Model file for the job. Use its own axes, mm. A direction names the side the tool comes from. Give positions to 0.01 mm unless a question says otherwise; leave off trailing zeros. Loops run counter-clockwise (first coordinate to the right, second up) from the corner with the lowest first, then second, coordinate; pieces in that order, holes last. Notation, with made-up numbers: M 81.25,45.5 L 134.25,45.5 A12 cw 134.25,66.5 Z; hole C 35.5,51.25 d8. An arc over 180 degrees is marked long. Answer in a Markdown table with one row per item.
```python
from build123d import *

# Parameters (mm, degrees)
SKETCH1_R           = 3.1
BOSS_EXTRUDE4_DEPTH = 13.7
SKETCH6_W           = 24.96
SKETCH6_H           = 31.16
CUT_EXTRUDE1_DEPTH  = 12.5
SKETCH7_W           = 19.96
SKETCH7_H           = 26.16
CUT_EXTRUDE2_DEPTH  = 12.5
SKETCH9_W           = 1.2
SKETCH9_H           = 12.5
CUT_EXTRUDE3_DEPTH  = 1.45
SKETCH10_W          = 1.2
SKETCH10_H          = 12.5
CUT_EXTRUDE4_DEPTH  = 1.45
CUT_EXTRUDE5_DEPTH  = 1.5
SKETCH12_W          = 7.5
SKETCH12_H          = 6
CUT_EXTRUDE6_DEPTH  = 20.892135624
BOSS_EXTRUDE5_DEPTH = 6
BOSS_EXTRUDE6_DEPTH = 7.7


with BuildPart() as part:
    # Sketch1 → Boss-Extrude4 (new body)
    with BuildSketch(Plane(origin=(0, 0, 0), x_dir=(1, 0, 0), z_dir=(0, 1, 0))):
        with BuildLine():
            Line((-1.559985024, 16.088570711), (-23.661955043, 33.271658997))
            ThreePointArc((-23.661955043, 33.271658997), (-29.74307331, 33.27087194), (-29.742286254, 27.189753673))
            Line((-29.742286254, 27.189753673), (-12.559985024, 5.088570711))
            Line((-12.559985024, 5.088570711), (-12.559985024, -6.971429289))
            Line((-12.559985024, -6.971429289), (-29.742286254, -29.072612251))
            ThreePointArc((-29.742286254, -29.072612251), (-29.74307331, -35.153730518), (-23.661955043, -35.154517574))
            Line((-23.661955043, -35.154517574), (-1.559985024, -17.971429289))
            Line((-1.559985024, -17.971429289), (4.300014976, -17.971429289))
            Line((4.300014976, -17.971429289), (26.401984994, -35.154517574))
            ThreePointArc((26.401984994, -35.154517574), (32.483103261, -35.153730518), (32.482316205, -29.072612251))
            Line((32.482316205, -29.072612251), (15.300014976, -6.971429289))
            Line((15.300014976, -6.971429289), (15.300014976, 5.088570711))
            Line((15.300014976, 5.088570711), (32.482316205, 27.189753673))
            ThreePointArc((32.482316205, 27.189753673), (32.483103261, 33.27087194), (26.401984994, 33.271658997))
            Line((26.401984994, 33.271658997), (4.300014976, 16.088570711))
            Line((4.300014976, 16.088570711), (-1.559985024, 16.088570711))
        make_face()
        with BuildLine():
            Line((15.300014976, -17.971429289), (15.300014976, -8.926547914))
            Line((15.300014976, -8.926547914), (30.013101167, -27.851638652))
            ThreePointArc((30.013101167, -27.851638652), (26.40152787, -29.073069325), (25.180248217, -32.684693693))
            Line((25.180248217, -32.684693693), (6.255121178, -17.971429289))
            Line((6.255121178, -17.971429289), (15.300014976, -17.971429289))
        make_face(mode=Mode.SUBTRACT)
        with Locations((-26.702120648, -32.113564912)):
            Circle(SKETCH1_R, mode=Mode.SUBTRACT)
        with BuildLine():
            Line((-12.559985024, -8.926547914), (-12.559985024, -17.971429289))
            Line((-12.559985024, -17.971429289), (-3.515091227, -17.971429289))
            Line((-3.515091227, -17.971429289), (-22.440218266, -32.684693693))
            ThreePointArc((-22.440218266, -32.684693693), (-23.661497919, -29.073069325), (-27.273071216, -27.851638652))
            Line((-27.273071216, -27.851638652), (-12.559985024, -8.926547914))
        make_face(mode=Mode.SUBTRACT)
        with BuildLine():
            Line((-3.515091227, 16.088570711), (-12.559985024, 16.088570711))
            Line((-12.559985024, 16.088570711), (-12.559985024, 7.043689336))
            Line((-12.559985024, 7.043689336), (-27.273071216, 25.968780075))
            ThreePointArc((-27.273071216, 25.968780075), (-23.661497919, 27.190210747), (-22.440218266, 30.801835115))
            Line((-22.440218266, 30.801835115), (-3.515091227, 16.088570711))
        make_face(mode=Mode.SUBTRACT)
        with Locations((-26.702120648, 30.230706335)):
            Circle(SKETCH1_R, mode=Mode.SUBTRACT)
        with BuildLine():
            Line((15.300014976, 7.043689336), (15.300014976, 16.088570711))
            Line((15.300014976, 16.088570711), (6.255121178, 16.088570711))
            Line((6.255121178, 16.088570711), (25.180248217, 30.801835115))
            ThreePointArc((25.180248217, 30.801835115), (26.40152787, 27.190210747), (30.013101167, 25.968780075))
            Line((30.013101167, 25.968780075), (15.300014976, 7.043689336))
        make_face(mode=Mode.SUBTRACT)
        with Locations((29.442150599, 30.230706335)):
            Circle(SKETCH1_R, mode=Mode.SUBTRACT)
        with Locations((29.442150599, -32.113564912)):
            Circle(SKETCH1_R, mode=Mode.SUBTRACT)
    extrude(amount=BOSS_EXTRUDE4_DEPTH)

    # Sketch6 → Cut-Extrude1 (cut)
    with BuildSketch(Plane(origin=(0, 13.7, 0), x_dir=(1, 0, 0), z_dir=(0, 1, 0))):
        with Locations((1.370014976, -0.941429289)):
            Rectangle(SKETCH6_W, SKETCH6_H)
    extrude(amount=-CUT_EXTRUDE1_DEPTH, mode=Mode.SUBTRACT)

    # Sketch7 → Cut-Extrude2 (cut)
    with BuildSketch(Plane(origin=(0, 1.2, 0), x_dir=(1, 0, 0), z_dir=(0, 1, 0))):
        with Locations((1.370014976, -0.941429289)):
            Rectangle(SKETCH7_W, SKETCH7_H)
    extrude(amount=-CUT_EXTRUDE2_DEPTH, mode=Mode.SUBTRACT)

    # Sketch9 → Cut-Extrude3 (cut)
    with BuildSketch(Plane.XY.offset(-14.638570711)):
        with Locations((-10.509985024, 7.45)):
            Rectangle(SKETCH9_W, SKETCH9_H)
        with Locations((13.250014976, 7.45)):
            Rectangle(SKETCH9_W, SKETCH9_H)
    extrude(amount=-CUT_EXTRUDE3_DEPTH, mode=Mode.SUBTRACT)

    # Sketch10 → Cut-Extrude4 (cut)
    with BuildSketch(Plane(origin=(0, 0, 16.521429289), x_dir=(-1, 0, 0), z_dir=(0, 0, -1))):
        with Locations((-13.250014976, 7.45)):
            Rectangle(SKETCH10_W, SKETCH10_H)
        with Locations((10.509985024, 7.45)):
            Rectangle(SKETCH10_W, SKETCH10_H)
    extrude(amount=-CUT_EXTRUDE4_DEPTH, mode=Mode.SUBTRACT)

    # Sketch11 → Cut-Extrude5 (cut)
    with BuildSketch(Plane.XZ):
        Polygon((-26.881022326, -29.561079875), (-26.032494188, -30.409608013), (-22.146132163, -26.523245987), (-22.9946603, -25.67471785), align=None)
        Polygon((24.886162114, -26.523245987), (25.734690251, -25.67471785), (29.621052277, -29.561079875), (28.772524139, -30.409608013), align=None)
        Polygon((29.621052277, 31.443938453), (28.772524139, 32.29246659), (24.886162114, 28.406104565), (25.734690251, 27.557576427), align=None)
        Polygon((-22.146132163, 28.406104565), (-22.9946603, 27.557576427), (-26.881022326, 31.443938453), (-26.032494188, 32.29246659), align=None)
    extrude(amount=-CUT_EXTRUDE5_DEPTH, mode=Mode.SUBTRACT)

    # Sketch12 → Cut-Extrude6 (cut, through all)
    with BuildSketch(Plane.XY.offset(-14.638570711)):
        with Locations((-2.379985024, 10.7)):
            Rectangle(SKETCH12_W, SKETCH12_H)
        with Locations((5.120014976, 10.7)):
            Rectangle(SKETCH12_W, SKETCH12_H)
    extrude(amount=-CUT_EXTRUDE6_DEPTH, mode=Mode.SUBTRACT)

    # Sketch14 → Boss-Extrude5 (add)
    with BuildSketch(Plane(origin=(0, 7.7, 0), x_dir=(1, 0, 0), z_dir=(0, 1, 0))):
        Polygon((-6.129985024, 19.641498953), (-6.129985024, 14.638570711), (-4.929985024, 14.638570711), (-4.929985024, 18.708563747), align=None)
        Polygon((8.870014976, 19.641498953), (8.870014976, 14.638570711), (7.62204126, 14.638570711), (7.62204126, 18.671266773), align=None)
    extrude(amount=BOSS_EXTRUDE5_DEPTH)

    # Sketch15 → Boss-Extrude6 (add)
    with BuildSketch(Plane.XZ.offset(-7.7)):
        Polygon((-6.129985024, -16.088570711), (-6.129985024, -18.121509447), (-3.515091227, -16.088570711), align=None)
        Polygon((8.870014976, -16.088570711), (8.870014976, -18.121509447), (6.255121178, -16.088570711), align=None)
    extrude(amount=BOSS_EXTRUDE6_DEPTH)


solid = part.part
```
Q1. Drop flat-ended pins along their axis: pin 1 (1.2 mm diameter, centred on y = 8, z = 17, fed in from -X); pin 2 (0.6 mm diameter, centred on y = 0.5, z = 1.5, fed in from -X); pin 3 (1.8 mm diameter, centred on x = 1, y = 10, fed in from +Z); pin 4 (6 mm diameter, centred on x = -10, z = 6, fed in from -Y). Give the stop position or say it passes through.
Reported:
| item | result |
|---|---|
| pin 1 | x = -20.82 |
| pin 2 | x = -12.56 |
| pin 3 | z = 17.97 |
| pin 4 | y = 0 |
Q2. Saw through at A-A (z = -1.5). Give the cut face in (x, y).
Reported:
| item | result |
|---|---|
| outline | M -12.56,0 L -8.61,0 L -8.61,1.2 L -11.11,1.2 L -11.11,13.7 L -12.56,13.7 Z; M 11.35,0 L 15.3,0 L 15.3,13.7 L 13.85,13.7 L 13.85,1.2 L 11.35,1.2 Z |
Q3. Saw through at D-D (y = 5.5). Give the number of separate pieces and of enclosed holes in the cut face, and give its area (3 significant figures).
Reported:
| item | result |
|---|---|
| separate pieces | 1 |
| enclosed holes | 5 |
| area | 527 mm² |
Q4. Mould opens along Z. For faces 6 (the face through (-23.745, 6.754, 31.182)), 7 (the face through (1.3, 7.7, -15.7)), 8 (the face through (15.196, 6.754, 26.443)) say: released by +Z, released by -Z, zero draft, split by the parting line, or undercut.
Reported:
| item | result |
|---|---|
| face 6 | undercut |
| face 7 | zero draft |
| face 8 | released by +Z |
Q5. 3-axis set-ups, long thin cutter, end or side, ignore diameter. For faces 1 (the face through (1, 13.7, 17)), 2 (the face through (-11.11, 7, 1)), 3 (the face through (-21.031, 6.754, 17.867)), 4 (the face through (-24, 1.5, 30)), 5 (the face through (-14.4, 6.75, -24.55)): which of +Z, -Z, +X, -X, +Y, -Y reach the whole face in a straight line?
Reported:
| item | result |
|---|---|
| face 1 | +Z, -Z, +X, -X, +Y |
| face 2 | +Y |
| face 3 | -X, +Y, -Y |
| face 4 | -Y |
| face 5 | +Y, -Y |
Q6. Probe probe 1 along X at (y, z) = (3.5, -14); probe 2 along Z at (x, y) = (-5.5, 1); probe 3 along X at (y, z) = (9.25, 17.5). List the from-to ranges inside material, lowest first.
Reported:
| item | result |
|---|---|
| probe 1 | -19.49 to -17.97, -12.56 to -11.11, 13.85 to 15.3, 20.71 to 22.23 |
| probe 2 | -19.15 to -12.14, 14.02 to 17.97, 19.51 to 21.03 |
| probe 3 | -20.75 to -19.23, -12.56 to -11.11, -9.91 to 12.65, 13.85 to 15.3, 21.97 to 23.49 |
Q7. Saw through at C-C (x = -21.5). Give the cut face in (y, z).
Reported:
| item | result |
|---|---|
| outline | M 0,-31.59 L 13.7,-31.59 L 13.7,-30.07 L 0,-30.07 Z; M 0,-18.54 L 13.7,-18.54 L 13.7,-16.59 L 0,-16.59 Z; M 0,18.47 L 13.7,18.47 L 13.7,20.43 L 0,20.43 Z; M 0,31.95 L 13.7,31.95 L 13.7,33.47 L 0,33.47 Z |
Q8. Saw through at B-B (z = 20.5). Give the cut face in (x, y), and give its area (3 significant figures).
Reported:
| item | result |
|---|---|
| outline | M -23.08,0 L -21.56,0 L -21.56,13.7 L -23.08,13.7 Z; M -6.77,0 L -4.81,0 L -4.81,13.7 L -6.77,13.7 Z; M 7.55,0 L 9.51,0 L 9.51,13.7 L 7.55,13.7 Z; M 24.3,0 L 25.82,0 L 25.82,13.7 L 24.3,13.7 Z |
| area | 95.2 mm² |
